from build123d import *

# Parameters (mm, degrees)
ESQUISSE3_R      = 2
ESQUISSE3_R_2    = 10
EXTRUSION2_DEPTH = 19
EXTRUSION4_DEPTH = 29


with BuildPart() as part:
    # Esquisse1 → Révolution1 (revolve)
    with BuildSketch(Plane.XY):
        Polygon((-6.5, 20), (-6.5, 44), (-8.5, 44), (-8.5, 22), (-11, 22), (-11, 0), (-10, 0), (-10, 20), align=None)
    revolve(axis=Axis((0, 0, 0), (0, 1, 0)))

    # Esquisse3 → Extrusion2 (add)
    with BuildSketch(Plane(origin=(0, 22, 0), x_dir=(1, 0, 0), z_dir=(0, 1, 0))):
        with BuildLine():
            Line((-11.313708499, -14), (-7.645328987, -14))
            Line((-7.645328987, -14), (-5.923372103, -9.268962344))
            ThreePointArc((-5.923372103, -9.268962344), (0.311535181, -10.995587562), (6.438678833, -8.918711504))
            Line((6.438678833, -8.918711504), (8.288116597, -14))
            Line((8.288116597, -14), (11.313708499, -14))
            ThreePointArc((11.313708499, -14), (12.727922061, -12.727922061), (14, -11.313708499))
            Line((14, -11.313708499), (14, -7.411373431))
            Line((14, -7.411373431), (9.388048674, -5.732760426))
            ThreePointArc((9.388048674, -5.732760426), (10.991831078, 0.423850851), (8.918711504, 6.438678833))
            Line((8.918711504, 6.438678833), (14, 8.288116597))
            Line((14, 8.288116597), (14, 11.313708499))
            ThreePointArc((14, 11.313708499), (12.727922061, 12.727922061), (11.313708499, 14))
            Line((11.313708499, 14), (7.690190806, 14))
            Line((7.690190806, 14), (5.959738542, 9.245621478))
            ThreePointArc((5.959738542, 9.245621478), (-0.112996861, 10.999419608), (-6.148420959, 9.12123455))
            Line((-6.148420959, 9.12123455), (-7.924146363, 14))
            Line((-7.924146363, 14), (-11.313708499, 14))
            ThreePointArc((-11.313708499, 14), (-12.727922061, 12.727922061), (-14, 11.313708499))
            Line((-14, 11.313708499), (-14, 7.924146363))
            Line((-14, 7.924146363), (-9.12123455, 6.148420959))
            ThreePointArc((-9.12123455, 6.148420959), (-11, 0), (-9.12123455, -6.148420959))
            Line((-9.12123455, -6.148420959), (-14, -7.924146363))
            Line((-14, -7.924146363), (-14, -11.313708499))
            ThreePointArc((-14, -11.313708499), (-12.727922061, -12.727922061), (-11.313708499, -14))
        make_face()
        with Locations((11, 11)):
            Circle(ESQUISSE3_R, mode=Mode.SUBTRACT)
        with Locations((-11, -11)):
            Circle(ESQUISSE3_R, mode=Mode.SUBTRACT)
        with Locations((-11, 11)):
            Circle(ESQUISSE3_R, mode=Mode.SUBTRACT)
        with Locations((11, -11)):
            Circle(ESQUISSE3_R, mode=Mode.SUBTRACT)
        Circle(ESQUISSE3_R_2, mode=Mode.SUBTRACT)
    extrude(amount=-EXTRUSION2_DEPTH)

    # Esquisse4 → Extrusion4 (cut, through all)
    with BuildSketch(Plane.XY.offset(14)):
        with BuildLine():
            Line((-1, 37), (-1, 12))
            ThreePointArc((-1, 12), (0, 11), (1, 12))
            Line((1, 12), (1, 37))
            ThreePointArc((1, 37), (0, 38), (-1, 37))
        make_face()
    extrude(amount=-EXTRUSION4_DEPTH, mode=Mode.SUBTRACT)


solid = part.part
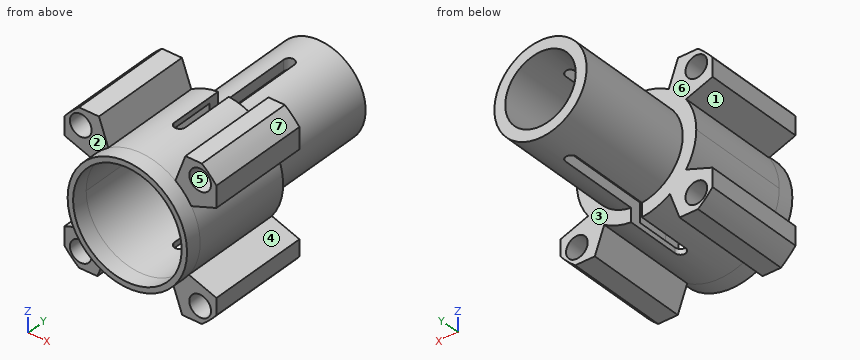
Read the model definition and answer for the solid it produces. Units are mm, in the model's axes. Face numbers are marked on the shaded views. A direction names the side the tool comes from. Round coordinates to 2 decimals unless told otherwise and drop trailing zeros. Write each loop counter-clockwise with the first axis right and the second up, starting at its lowest first coordinate (ties: lowest second). Pieces come first, ordered by that corner, then holes.
Q1. Find section B-B on y = 10.5. State how many separate pieces and enclosed holes the cut face has, and give its area (3 significant figures).
Values:
separate pieces: 1
enclosed holes: 5
area: 196 mm2
Q2. The mould has two halves that part along Z. Classify the marked faces 5, 6 and 7: released by +Z, released by -Z, zero draft, split by the parting line, or undercut.
Values:
face 5: undercut
face 6: zero draft
face 7: released by +Z
Q3. Find section A-A on x = 5.25. Determine the outline of the cut face in (y, z).
Values:
outline: (0, -9.67) - (22, -9.67) - (22, -6.68) - (44, -6.68) - (44, -3.83) - (20, -3.83) - (20, -8.51) - (0, -8.51) - close; (0, 8.51) - (20, 8.51) - (20, 3.83) - (44, 3.83) - (44, 6.68) - (22, 6.68) - (22, 9.67) - (0, 9.67) - close
Q4. Flat-ended cylindrical pins translate along their axes: P1, Ø3.5, axis at y = 27.5, z = 9, coming from the +X side; P2, Ø4.5, axis at x = -3.5, z = 5, coming from the -Y side; P3, Ø5, axis at x = 11, z = 11, coming from the +Y side; P4, Ø4, axis at x = -2.5, z = 0.5, coming from the -Y side. Find the tip coordinate at first contact, or state that the pin passes through.
Values:
P1: stops at x = 4.44
P2: stops at y = 20
P3: stops at y = 22
P4: passes through
Q5. A tool of negligible diameter and unlimited length cuts with its end or side. For the marked faces 1, 2, 3 and 4, from which of +Z, -Z, +X, -X, +Y, -Y can it reach the whole face along a straight path? Write none if from no direction.
Values:
face 1: -X, +Y, -Y
face 2: +Z, -X, -Y
face 3: +X, +Y
face 4: +X, +Y, -Y
Q6. Straight lines are drawn through the part: line 1 (X direction, y = 31.5, z = 0); line 2 (Z direction, x = 0, y = 2.35); line 3 (X direction, y = 14.5, z = 11). For each, find the intervals that lie inside material, in ascending order.
Values:
line 1: x = -8.5 to -6.5, 6.5 to 8.5
line 2: z = -11 to -10, 10 to 11
line 3: x = -14 to -13, -9 to -6.55, 7.2 to 9, 13 to 14
Q7. Find section C-C on z = -3.75. Determine the outline of the cut face in (x, y), and give its area (3 significant figures).
Values:
outline: (-10.34, 0) - (-9.27, 0) - (-9.27, 20) - (-5.31, 20) - (-5.31, 44) - (-7.63, 44) - (-7.63, 22) - (-10.34, 22) - close; (5.31, 20) - (9.27, 20) - (9.27, 0) - (10.34, 0) - (10.34, 22) - (7.63, 22) - (7.63, 44) - (5.31, 44) - close
area: 165 mm2
